```python
from build123d import *

# Parameters (mm, degrees)
F0_W     = 150
F0_H     = 150
F0_R     = 4.675
F0_R_2   = 4.025
F1_DEPTH = 14.45
F2_DEPTH = 25
F3_DEPTH = 5.55


with BuildPart() as f1:
    # F0 (on Top) → F1 (new body)
    with BuildSketch(Plane.XY):
        with Locations((-75, 75)):
            Rectangle(F0_W, F0_H)
        with Locations((-120, 30)):
            Circle(F0_R, mode=Mode.SUBTRACT)
        with Locations((-90, 30)):
            Circle(F0_R, mode=Mode.SUBTRACT)
        with Locations((-120, 60)):
            Circle(F0_R, mode=Mode.SUBTRACT)
        with Locations((-90, 60)):
            Circle(F0_R, mode=Mode.SUBTRACT)
        with Locations((-60, 30)):
            Circle(F0_R, mode=Mode.SUBTRACT)
        with Locations((-30, 30)):
            Circle(F0_R, mode=Mode.SUBTRACT)
        with Locations((-60, 60)):
            Circle(F0_R, mode=Mode.SUBTRACT)
        with Locations((-30, 60)):
            Circle(F0_R, mode=Mode.SUBTRACT)
        with Locations((-120, 90)):
            Circle(F0_R, mode=Mode.SUBTRACT)
        with Locations((-90, 90)):
            Circle(F0_R, mode=Mode.SUBTRACT)
        with Locations((-120, 120)):
            Circle(F0_R, mode=Mode.SUBTRACT)
        with Locations((-90, 120)):
            Circle(F0_R, mode=Mode.SUBTRACT)
        with Locations((-60, 90)):
            Circle(F0_R, mode=Mode.SUBTRACT)
        with Locations((-30, 90)):
            Circle(F0_R, mode=Mode.SUBTRACT)
        with Locations((-60, 120)):
            Circle(F0_R, mode=Mode.SUBTRACT)
        with Locations((-30, 120)):
            Circle(F0_R, mode=Mode.SUBTRACT)
        with Locations((-120, 120)):
            Circle(F0_R)
        with Locations((-120, 120)):
            Circle(F0_R_2, mode=Mode.SUBTRACT)
        with Locations((-90, 120)):
            Circle(F0_R)
        with Locations((-90, 120)):
            Circle(F0_R_2, mode=Mode.SUBTRACT)
        with Locations((-90, 90)):
            Circle(F0_R)
        with Locations((-90, 90)):
            Circle(F0_R_2, mode=Mode.SUBTRACT)
        with Locations((-60, 120)):
            Circle(F0_R)
        with Locations((-60, 120)):
            Circle(F0_R_2, mode=Mode.SUBTRACT)
        with Locations((-60, 90)):
            Circle(F0_R)
        with Locations((-60, 90)):
            Circle(F0_R_2, mode=Mode.SUBTRACT)
        with Locations((-120, 90)):
            Circle(F0_R)
        with Locations((-120, 90)):
            Circle(F0_R_2, mode=Mode.SUBTRACT)
        with Locations((-30, 120)):
            Circle(F0_R)
        with Locations((-30, 120)):
            Circle(F0_R_2, mode=Mode.SUBTRACT)
        with Locations((-30, 90)):
            Circle(F0_R)
        with Locations((-30, 90)):
            Circle(F0_R_2, mode=Mode.SUBTRACT)
        with Locations((-120, 60)):
            Circle(F0_R)
        with Locations((-120, 60)):
            Circle(F0_R_2, mode=Mode.SUBTRACT)
        with Locations((-90, 60)):
            Circle(F0_R)
        with Locations((-90, 60)):
            Circle(F0_R_2, mode=Mode.SUBTRACT)
        with Locations((-90, 30)):
            Circle(F0_R)
        with Locations((-90, 30)):
            Circle(F0_R_2, mode=Mode.SUBTRACT)
        with Locations((-120, 30)):
            Circle(F0_R)
        with Locations((-120, 30)):
            Circle(F0_R_2, mode=Mode.SUBTRACT)
        with Locations((-60, 30)):
            Circle(F0_R)
        with Locations((-60, 30)):
            Circle(F0_R_2, mode=Mode.SUBTRACT)
        with Locations((-30, 30)):
            Circle(F0_R)
        with Locations((-30, 30)):
            Circle(F0_R_2, mode=Mode.SUBTRACT)
        with Locations((-60, 60)):
            Circle(F0_R)
        with Locations((-60, 60)):
            Circle(F0_R_2, mode=Mode.SUBTRACT)
        with Locations((-30, 60)):
            Circle(F0_R)
        with Locations((-30, 60)):
            Circle(F0_R_2, mode=Mode.SUBTRACT)
        with Locations((-120, 120)):
            Circle(F0_R_2)
        with Locations((-90, 120)):
            Circle(F0_R_2)
        with Locations((-60, 120)):
            Circle(F0_R_2)
        with Locations((-30, 90)):
            Circle(F0_R_2)
        with Locations((-60, 90)):
            Circle(F0_R_2)
        with Locations((-90, 90)):
            Circle(F0_R_2)
        with Locations((-120, 60)):
            Circle(F0_R_2)
        with Locations((-90, 60)):
            Circle(F0_R_2)
        with Locations((-60, 60)):
            Circle(F0_R_2)
        with Locations((-30, 60)):
            Circle(F0_R_2)
        with Locations((-30, 30)):
            Circle(F0_R_2)
        with Locations((-60, 30)):
            Circle(F0_R_2)
        with Locations((-90, 30)):
            Circle(F0_R_2)
        with Locations((-120, 90)):
            Circle(F0_R_2)
        with Locations((-30, 120)):
            Circle(F0_R_2)
        with Locations((-120, 30)):
            Circle(F0_R_2)
    extrude(amount=F1_DEPTH)

    # F0 (on Top) → F2 (cut)
    with BuildSketch(Plane.XY):
        with Locations((-120, 30)):
            Circle(F0_R_2)
        with Locations((-90, 30)):
            Circle(F0_R_2)
        with Locations((-60, 30)):
            Circle(F0_R_2)
        with Locations((-30, 30)):
            Circle(F0_R_2)
        with Locations((-30, 60)):
            Circle(F0_R_2)
        with Locations((-60, 60)):
            Circle(F0_R_2)
        with Locations((-90, 60)):
            Circle(F0_R_2)
        with Locations((-120, 60)):
            Circle(F0_R_2)
        with Locations((-120, 90)):
            Circle(F0_R_2)
        with Locations((-90, 90)):
            Circle(F0_R_2)
        with Locations((-60, 90)):
            Circle(F0_R_2)
        with Locations((-30, 90)):
            Circle(F0_R_2)
        with Locations((-30, 120)):
            Circle(F0_R_2)
        with Locations((-60, 120)):
            Circle(F0_R_2)
        with Locations((-90, 120)):
            Circle(F0_R_2)
        with Locations((-120, 120)):
            Circle(F0_R_2)
    extrude(amount=F2_DEPTH, mode=Mode.SUBTRACT)

    # F0 (on Top) → F3 (cut)
    with BuildSketch(Plane.XY):
        with Locations((-120, 30)):
            Circle(F0_R)
        with Locations((-120, 30)):
            Circle(F0_R_2, mode=Mode.SUBTRACT)
        with Locations((-90, 30)):
            Circle(F0_R)
        with Locations((-90, 30)):
            Circle(F0_R_2, mode=Mode.SUBTRACT)
        with Locations((-60, 30)):
            Circle(F0_R)
        with Locations((-60, 30)):
            Circle(F0_R_2, mode=Mode.SUBTRACT)
        with Locations((-30, 30)):
            Circle(F0_R)
        with Locations((-30, 30)):
            Circle(F0_R_2, mode=Mode.SUBTRACT)
        with Locations((-30, 60)):
            Circle(F0_R)
        with Locations((-30, 60)):
            Circle(F0_R_2, mode=Mode.SUBTRACT)
        with Locations((-60, 60)):
            Circle(F0_R)
        with Locations((-60, 60)):
            Circle(F0_R_2, mode=Mode.SUBTRACT)
        with Locations((-90, 60)):
            Circle(F0_R)
        with Locations((-90, 60)):
            Circle(F0_R_2, mode=Mode.SUBTRACT)
        with Locations((-120, 60)):
            Circle(F0_R)
        with Locations((-120, 60)):
            Circle(F0_R_2, mode=Mode.SUBTRACT)
        with Locations((-120, 90)):
            Circle(F0_R)
        with Locations((-120, 90)):
            Circle(F0_R_2, mode=Mode.SUBTRACT)
        with Locations((-90, 90)):
            Circle(F0_R)
        with Locations((-90, 90)):
            Circle(F0_R_2, mode=Mode.SUBTRACT)
        with Locations((-60, 90)):
            Circle(F0_R)
        with Locations((-60, 90)):
            Circle(F0_R_2, mode=Mode.SUBTRACT)
        with Locations((-30, 90)):
            Circle(F0_R)
        with Locations((-30, 90)):
            Circle(F0_R_2, mode=Mode.SUBTRACT)
        with Locations((-30, 120)):
            Circle(F0_R)
        with Locations((-30, 120)):
            Circle(F0_R_2, mode=Mode.SUBTRACT)
        with Locations((-60, 120)):
            Circle(F0_R)
        with Locations((-60, 120)):
            Circle(F0_R_2, mode=Mode.SUBTRACT)
        with Locations((-90, 120)):
            Circle(F0_R)
        with Locations((-90, 120)):
            Circle(F0_R_2, mode=Mode.SUBTRACT)
        with Locations((-120, 120)):
            Circle(F0_R)
        with Locations((-120, 120)):
            Circle(F0_R_2, mode=Mode.SUBTRACT)
    extrude(amount=F3_DEPTH, mode=Mode.SUBTRACT)


solid = f1.part
```
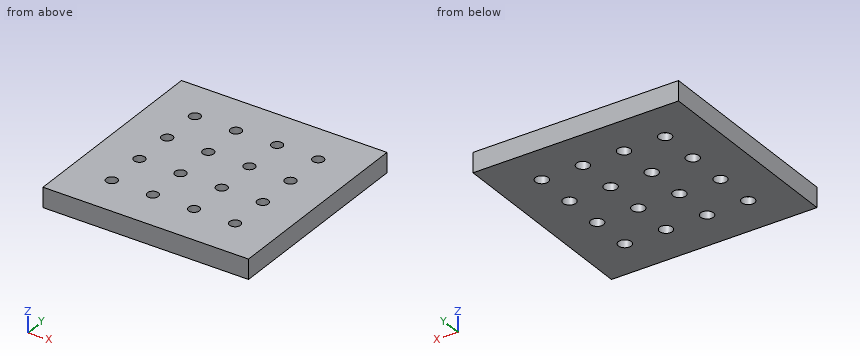
Could you check a few things on this model? Use its own coordinates, in mm. Give positions to 0.01 mm unless a question says otherwise; leave off trailing zeros.
Q1. If I drill on line 1 along Y through (x, z) = (-120, 3.1) (3 decimals); line 2 along Y through (x, z) = (-90, 8.5) (3 decimals), over which ranges is the centre line in solid material (lowest first)?
Q2. Suppose I cut it at A-A, the plane z = 9. Count the separate pieces of the cut face and the enclosed holes in it, and give its area (3 significant figures).
Q3. I'm going to push flat-ended pins straight in: P1, Ø4.5, axis at x = -91.5, y = 28.5, coming from the -Z side; P2, Ø5.5, axis at x = -90, y = 120, coming from the +Z side. Where does each tip first touch, or does it pass through?
Solution:
1. line 1: y = 0 to 25.325, 34.675 to 55.325, 64.675 to 85.325, 94.675 to 115.325, 124.675 to 150
1. line 2: y = 0 to 25.975, 34.025 to 55.975, 64.025 to 85.975, 94.025 to 115.975, 124.025 to 150
2. separate pieces: 1
2. enclosed holes: 16
2. area: 21,700 mm2
3. P1: stops at z = 5.55
3. P2: passes through
